Autodesk Fusion 360 part; units mm, degrees
sketch "Sketch1" plane through (0, 0, 0) normal (1, 0, 0) x (0, 1, 0)
  circle A0 centre (0, 0) radius 0.5
  line L0 (0.325, -0.325) -> (-0.325, -0.325)
  line L1 (-0.325, -0.325) -> (-0.325, 0.325)
  line L2 (-0.325, 0.325) -> (0.325, 0.325)
  line L3 (0.325, 0.325) -> (0.325, -0.325)
  line L4 (0.325, -0.325) -> (-0.325, 0.325) construction
  line L5 (-0.325, -0.325) -> (0.325, 0.325) construction
  dimension "d1" = 1
  dimension "d2" = 0.65
  dimension "d3" = 0.65
extrude "Extrude1" add sketch "Sketch1" along normal blind 40 contours A0 | L0 L1 L2 L3
sketch "Sketch2" plane through (40, 0, 0) normal (1, 0, 0) x (0, 1, 0)
  circle A0 centre (0, 0) radius 0.5
  line L0 (0.325, -0.325) -> (-0.325, -0.325)
  line L1 (-0.325, -0.325) -> (-0.325, 0.325)
  line L2 (-0.325, 0.325) -> (0.325, 0.325)
  line L3 (0.325, 0.325) -> (0.325, -0.325)
  line L4 (0.325, -0.325) -> (-0.325, 0.325) construction
  line L5 (-0.325, -0.325) -> (0.325, 0.325) construction
  dimension "d8" = 0.65
  dimension "d9" = 0.65
extrude "Extrude2" add sketch "Sketch2" along normal blind 1.915 contours L0 L1 L2 L3
extrude "Extrude3" add sketch "Sketch1" against normal blind 1.915 contours L0 L1 L2 L3
sketch "Sketch3" plane through (0, 0, -0.325) normal (0, 0, -1) x (1, 0, 0)
  line L0 (40, 0.325) -> (40, -0.325)
  line L1 (40, -0.325) -> (41.915, -0.325)
  line L2 (41.915, -0.325) -> (41.915, 0.325)
  line L3 (41.915, 0.325) -> (40, 0.325)
  line L4 (41.915, 0.325) -> (41.265, 0.325)
  line L5 (41.265, 0.325) -> (41.265, -0.325)
  line L6 (41.265, -0.325) -> (41.915, -0.325)
  line L7 (41.915, -0.325) -> (41.915, 0.325)
  line L8 (41.915, 0.325) -> (41.265, -0.325) construction
  line L9 (41.265, 0.325) -> (41.915, -0.325) construction
  point P0 (41.59, 0)
  dimension "d14" = 0.65
  dimension "d15" = 0.65
sketch "Sketch4" plane through (0, 0, -0.325) normal (0, 0, -1) x (1, 0, 0)
  line L0 (0, -0.325) -> (0, 0.325)
  line L1 (0, 0.325) -> (-1.915, 0.325)
  line L2 (-1.915, 0.325) -> (-1.915, -0.325)
  line L3 (-1.915, -0.325) -> (0, -0.325)
  line L4 (-1.265, -0.325) -> (-1.915, -0.325)
  line L5 (-1.915, -0.325) -> (-1.915, 0.325)
  line L6 (-1.915, 0.325) -> (-1.265, 0.325)
  line L7 (-1.265, 0.325) -> (-1.265, -0.325)
  line L8 (-1.265, -0.325) -> (-1.915, 0.325) construction
  line L9 (-1.915, -0.325) -> (-1.265, 0.325) construction
  point P0 (-1.59, 0)
  dimension "d17" = 0.65
  dimension "d18" = 0.65
extrude "Extrude4" add sketch "Sketch4" sketch "Sketch3" along normal blind 2.75 contours L1 L2 L3 L4 L5 L6 L7 of sketch 2 contours L1 L2 L3 L4 L5 L6 L7
fillet "Fillet1" radius 0.5 2 edges at (-1.265, 0, -0.325) (41.265, 0, -0.325)
fillet "Fillet2" radius 1 2 edges at (-1.915, 0, 0.325) (41.915, 0, 0.325)
fillet "Fillet3" radius 0.2 28 edges at (-1.59, -0.325, -3.075) (-1.265, 0, -3.075) (-1.59, 0.325, -3.075) (-1.915, 0, -3.075) (-1.1186, -0.325, -0.4714) (-1.265, -0.325, -1.95) (-0.4575, -0.325, 0.325) (-1.6221, -0.325, 0.0321) (-1.915, -0.325, -1.875) (-0.4575, 0.325, 0.325) (-1.6221, 0.325, 0.0321) (-1.915, 0.325, -1.875) (-1.1186, 0.325, -0.4714) (-1.265, 0.325, -1.95) (40.4575, -0.325, 0.325) (41.6221, -0.325, 0.0321) (41.915, -0.325, -1.875) (41.265, -0.325, -1.95) (41.1186, -0.325, -0.4714) (41.915, 0.325, -1.875) (41.6221, 0.325, 0.0321) (40.4575, 0.325, 0.325) (41.1186, 0.325, -0.4714) (41.265, 0.325, -1.95) (41.59, 0.325, -3.075) (41.915, 0, -3.075) (41.59, -0.325, -3.075) (41.265, 0, -3.075)
equation "d1 = width"
equation "d2 = d3"
equation "d3 = d1 * 0.65"
equation "width = 1 mm"
equation "baseLenght = 40 mm"
equation "d6 = baseLenght"
equation "d8 = width * 0.65"
equation "d9 = d8"
equation "d14 = width * 0.65"
equation "d15 = d14"
equation "d17 = width * 0.65"
equation "d18 = d17"
equation "d26 = 0.2 * width"
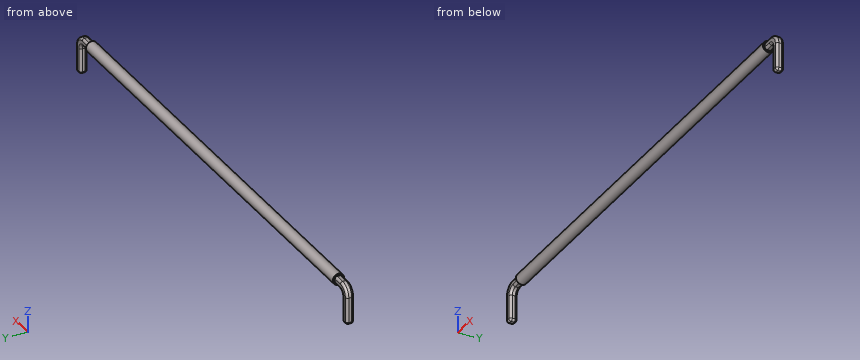
Part model, mm, in its own coordinate system. Coordinates: 2 decimals unless noted, no trailing zeros. Write each loop counter-clockwise with the first axis right and the second up, starting at its lowest first coordinate (ties: lowest second). Pieces come first, ordered by that corner, then holes.
Item 1: Slice it at B-B (x = 37). Write the cut outline in (y, z), and give its area (3 significant figures).
Item 2: Probe line 1 (X direction, y = 0, z = -2.05) (3 decimals); line 2 (X direction, y = -0.4, z = 0.2); line 3 (X direction, y = -0.05, z = -0.6). List the from-to ranges inside material, lowest first.
Item 3: Pin check, flat tips, straight feed: pin 1 (0.5 mm diameter, centred on y = 0, z = 0, fed in from -X); pin 2 (0.9 mm diameter, centred on x = 41, z = -1, fed in from -Y). Stop position of each tip, or through.
Item 4: Slice it at A-A (z = -1.55). Write the cut outline in (x, y) (3 decimals), and give its area (3 significant figures).
Results found:
1. outline: circle Ø1 at (0, 0)
1. area: 0.785 mm2
2. line 1: x = -1.915 to -1.265, 41.265 to 41.915
2. line 2: x = 0 to 40
2. line 3: x = -1.91 to -1.21, 41.21 to 41.91
3. pin 1: stops at x = -1.82
3. pin 2: stops at y = -0.32
4. outline: (-1.915, -0.125) arc R0.2 ccw to (-1.715, -0.325) - (-1.465, -0.325) arc R0.2 ccw to (-1.265, -0.125) - (-1.265, 0.125) arc R0.2 ccw to (-1.465, 0.325) - (-1.715, 0.325) arc R0.2 ccw to (-1.915, 0.125) - close; (41.265, -0.125) arc R0.2 ccw to (41.465, -0.325) - (41.715, -0.325) arc R0.2 ccw to (41.915, -0.125) - (41.915, 0.125) arc R0.2 ccw to (41.715, 0.325) - (41.465, 0.325) arc R0.2 ccw to (41.265, 0.125) - close
4. area: 0.776 mm2
